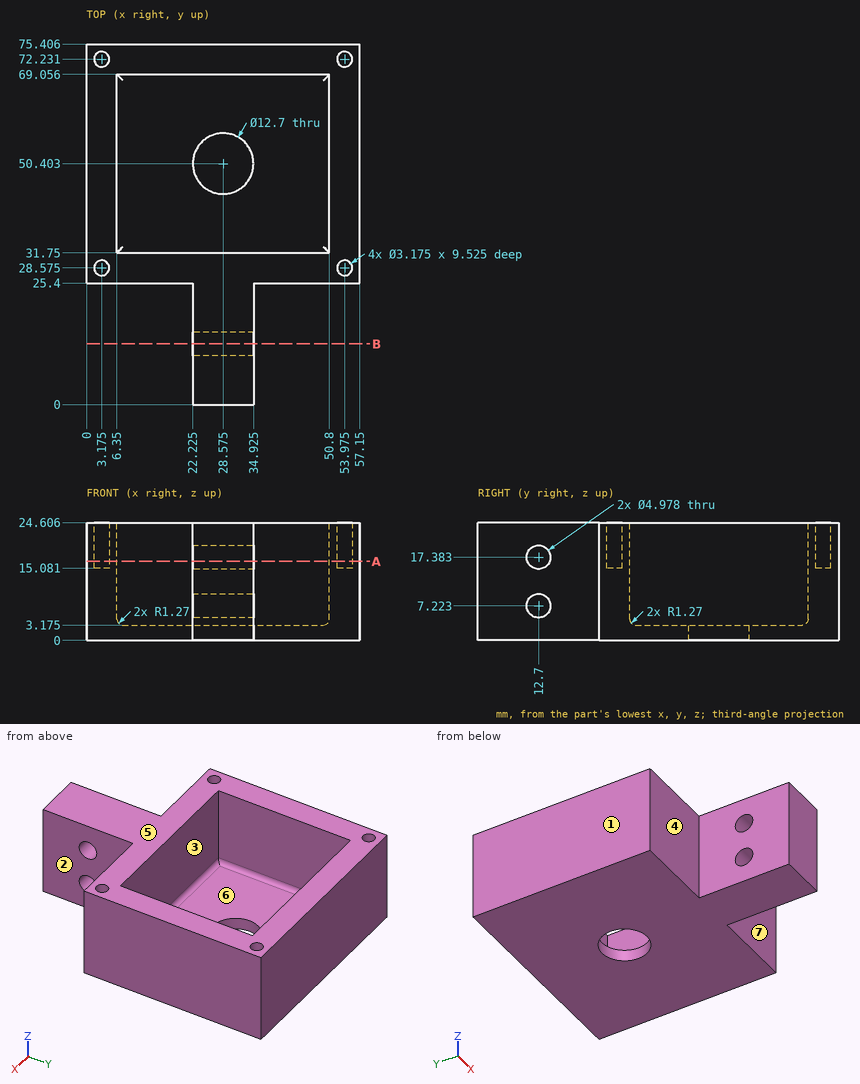
Design review of the part shown in the three views and the two pictorial views. Dimensions are in mm from the part's minimum x, y and z. A direction names the side the tool comes from. Round coordinates to 2 decimals unless told otherwise and drop trailing zeros. Loops run counter-clockwise (first coordinate to the right, second up) from the corner with the lowest first, then second, coordinate; pieces in that order, holes last. Notation, with made-up numbers: M 19,29.25 L 62,29.25 A26 ccw 62,46.25 Z; hole C 21.5,45.25 d10. An arc over 180 degrees is marked long. Write item = value, one per line.
Item 1: The part is to be moulded in two halves that separate along Y. For the marked faces 5, 6 and 7, say which applies: released by +Y, released by -Y, zero draft, split by the parting line, or undercut.
Return value:
face_5 = zero draft
face_6 = undercut
face_7 = released by -Y
Item 2: For line 1 (Y direction, x = 14, z = 22.5); line 2 (Y direction, x = 34.5, z = 23.25); line 3 (X direction, y = 57.5, z = 6.5), list the stretches that pass through material, from the lowest coordinate up. Write a range as [from, to].
Return value:
line_1 = [25.4, 31.75], [69.06, 75.41]
line_2 = [0, 31.75], [69.06, 75.41]
line_3 = [0, 6.35], [50.8, 57.15]
Item 3: Insertion check: P1, Ø7.5, axis at y = 14, z = 15.5, coming from the +X side (3 decimals); P2, Ø6, axis at x = 38.5, z = 17, coming from the -Y side; P3, Ø17.5, axis at x = 27.5, y = 49.5, coming from the +Z side (3 decimals); P4, Ø4, axis at y = 12.7, z = 17.38, coming from the -X side. Each pin has a flat end and moves straight along its axis. Give the tip position at first contact, or say it passes through.
Return value:
P1 = 34.925
P2 = 25.4
P3 = 3.175
P4 = through
Item 4: Take a section at B-B on y = 12.7. Write out the cut boundary in (x, z) (1 decimal), then the cut area to 3 significant figures.
Return value:
outline = M 22.2,0 L 34.9,0 L 34.9,4.7 L 22.2,4.7 Z; M 22.2,9.7 L 34.9,9.7 L 34.9,14.9 L 22.2,14.9 Z; M 22.2,19.9 L 34.9,19.9 L 34.9,24.6 L 22.2,24.6 Z
area = 186 mm2
Item 5: Take a section at A-A on z = 16.5. State how many separate pieces and enclosed holes the cut face has, then the cut area to 3 significant figures.
Return value:
separate_pieces = 2
enclosed_holes = 5
area = 1,430 mm2
Item 6: Machinability: for the marked faces 1, 2, 3 and 4, which of the approach directions +Z, -Z, +X, -X, +Y, -Y give a long, thin tool a straight path to every point of the face, cutting with its end or side? Answer none if there is none.
Return value:
face_1 = +Z, -Z, -X, +Y, -Y
face_2 = +Z, -Z, +X, -Y
face_3 = +Z
face_4 = +Z, -Z, -X, -Y
